```python
from build123d import *

# Parameters (mm, degrees)
SKETCH1_W           = 150
SKETCH1_H           = 150
BOSS_EXTRUDE1_DEPTH = 1250
SKETCH2_R           = 5
BOLTS_DEPTH         = 1262.199825563
TOPCUT_DEPTH        = 1262.199825563
ROOFCUT_DEPTH       = 1262.199825563
CUT_EXTRUDE4_DEPTH  = 1262.199825563
SKETCH6_R           = 5
CUT_EXTRUDE5_DEPTH  = 1262.199825563
CUT_EXTRUDE6_DEPTH  = 50


with BuildPart() as part:
    # Sketch1 → Boss-Extrude1 (new, symmetric)
    with BuildSketch(Plane(origin=(0, 0, 0), x_dir=(1, 0, 0), z_dir=(0, 1, 0))):
        Rectangle(SKETCH1_W, SKETCH1_H)
    extrude(amount=BOSS_EXTRUDE1_DEPTH, both=True)

    # Sketch2 → Bolts (cut, through all)
    with BuildSketch(Plane.XY.offset(75)):
        with Locations((0, 810)):
            Circle(SKETCH2_R)
        with Locations((0, -370)):
            Circle(SKETCH2_R)
    extrude(amount=-BOLTS_DEPTH, mode=Mode.SUBTRACT)

    # Sketch3 → TopCut (cut, through all)
    with BuildSketch(Plane.XY.offset(75)):
        Polygon((-75, 1068.159196847), (-20.84827249, 984.090234633), (-75, 949.20923319), align=None)
    extrude(amount=-TOPCUT_DEPTH, mode=Mode.SUBTRACT)

    # Sketch4 → RoofCut (cut, through all)
    with BuildSketch(Plane.XY.offset(75)):
        Polygon((75, 1250), (-75, 1215.956662981), (-75, 1250), align=None)
    extrude(amount=-ROOFCUT_DEPTH, mode=Mode.SUBTRACT)

    # Sketch5 → Cut-Extrude4 (cut, through all)
    with BuildSketch(Plane.XY.offset(75)):
        Polygon((75, -1159.47022319), (-65.544812434, -1250), (75, -1250), align=None)
    extrude(amount=-CUT_EXTRUDE4_DEPTH, mode=Mode.SUBTRACT)

    # Sketch6 → Cut-Extrude5 (cut, through all)
    with BuildSketch(Plane.ZY.offset(75)):
        with Locations((0, 250)):
            Circle(SKETCH6_R)
    extrude(amount=-CUT_EXTRUDE5_DEPTH, mode=Mode.SUBTRACT)

    # Sketch7 → Cut-Extrude6 (cut)
    with BuildSketch(Plane(origin=(0, 0, -75), x_dir=(-1, 0, 0), z_dir=(0, 0, -1))):
        Polygon((-75, 665.302341615), (75.500489844, 771.478930046), (75, 954.697658385), (-75, 848.874160527), align=None)
    extrude(amount=-CUT_EXTRUDE6_DEPTH, mode=Mode.SUBTRACT)


solid = part.part
```
Read the model definition and answer for the solid it produces. Units are mm, in the model's axes. A direction names the side the tool comes from. Coordinates: 2 decimals unless noted, no trailing zeros. Loops run counter-clockwise (first coordinate to the right, second up) from the corner with the lowest first, then second, coordinate; pieces in that order, holes last.
(1) The part is cut by section B-B (x = 26.5). Determine the outline of the cut face in (y, z), and give its area (3 significant figures).
Solution:
outline: (-1190.71, -75) - (699.52, -75) - (699.52, -25) - (883.09, -25) - (883.09, -75) - (1238.99, -75) - (1238.99, 75) - (-1190.71, 75) - close; hole circle Ø10 at (250, 0)
area: 355,000 mm2
(2) Flat-ended cylindrical pins translate along their axes: pin 1 Ø6 at (x, z) = (2.5, 42.5) entering from +Y; pin 2 Ø10 at (x, z) = (-35, -47.5) entering from +Y; pin 3 Ø2 at (x, z) = (-34.5, 39) entering from -Y; pin 4 Ø11.5 at (y, z) = (250, 0) entering from -X. Find the tip coordinate at first contact, or state that the pin passes through.
Solution:
pin 1: stops at y = 1234.23
pin 2: stops at y = 1226.17
pin 3: stops at y = -1230.65
pin 4: stops at x = -75
(3) The part is cut by section A-A (z = 43). Determine the outline of the cut face in (x, y).
Solution:
outline: (-75, -1250) - (-65.54, -1250) - (75, -1159.47) - (75, 1250) - (-75, 1215.96) - (-75, 1068.16) - (-20.85, 984.09) - (-75, 949.21) - close; hole circle Ø10 at (0, -370); hole circle Ø10 at (0, 810)
(4) The mould has two halves that part along Y. Classify faces 1 (the face through (1.05, 1233.217, 1.05)), 2 (the face through (-47.55, 966.89, 1.05)), 3 (the face through (-1, -225, -75)): released by +Y, released by -Y, zero draft, split by the parting line, or undercut.
Solution:
face 1: released by +Y
face 2: undercut
face 3: zero draft
(5) A tool of negligible diameter and unlimited length cuts with its end or side. For faces 4 (the face through (18, 811, -25)), 5 (the face through (1.012, 901.072, -50.35)), 6 (the face through (1.05, 717.473, -50.35)), 7 (the face through (-48.3, 1026.71, 1.05)), from which of +Z, -Z, +X, -X, +Y, -Y can it reach the whole face along a straight path? Write none if from no direction.
Solution:
face 4: -Z
face 5: -Z, -X
face 6: -Z, +X
face 7: +Z, -Z, -X
(6) Consider line 1 along X through (y, z) = (-370, -28); line 2 along Y through (x, z) = (0, 49.5); line 3 along Y through (x, z) = (0, -26). Determine where each line is inside the solid, lowest interval first.
Solution:
line 1: x = -75 to -5, 5 to 75
line 2: y = -1207.78 to -375, -365 to 805, 815 to 1232.98
line 3: y = -1207.78 to -375, -365 to 718.21, 901.79 to 1232.98
